Geometry: see drawing. Coordinates: mm, zero at the bounding-box minimum. A direction names the side the tool comes from. Coordinates: 2 decimals unless noted, no trailing zeros. Order: outer loops, then holes, each group sorted by start corner. A loop starts at its lowest first (then second) coordinate and runs counter-clockwise, first axis right, second up.
Item 1: Section D-D on y = 18. Return the cut outline in (x, z).
Item 2: Ray query, line 1 (Y direction, x = 15, z = 3); line 2 (X direction, y = 25.5, z = 16.5); line 3 (Z direction, x = 81, y = 4). Return the intervals inside material, ascending.
Item 3: Mould query, pull axis X, two halves, no side actions, for the marked faces 5, 6 and 7. Classes: released by +X, released by -X, zero draft, split by the parting line, or undercut.
Item 4: Contact query for flat-ended pins moving along their axis: P1, Ø2, axis at y = 6, z = 28.5, coming from the +X side; P2, Ø10.5, axis at x = 15, y = 29, coming from the +Z side; P3, Ø2, axis at y = 30, z = 34.5, coming from the +X side. Output: stop coordinate, or through.
Item 5: Section A-A on y = 10. Return the cut outline in (x, z).
Item 6: Section B-B on z = 9. Return the cut outline in (x, y), then the cut area to 3 significant figures.
Item 7: Section C-C on x = 15. Return the cut outline in (y, z).
Item 8: Reachability of the marked faces 1, 2, 3 and 4 from +Z, -Z, +X, -X, +Y, -Y: full face, straight path, thin tool, end or side. Return the list, or none.
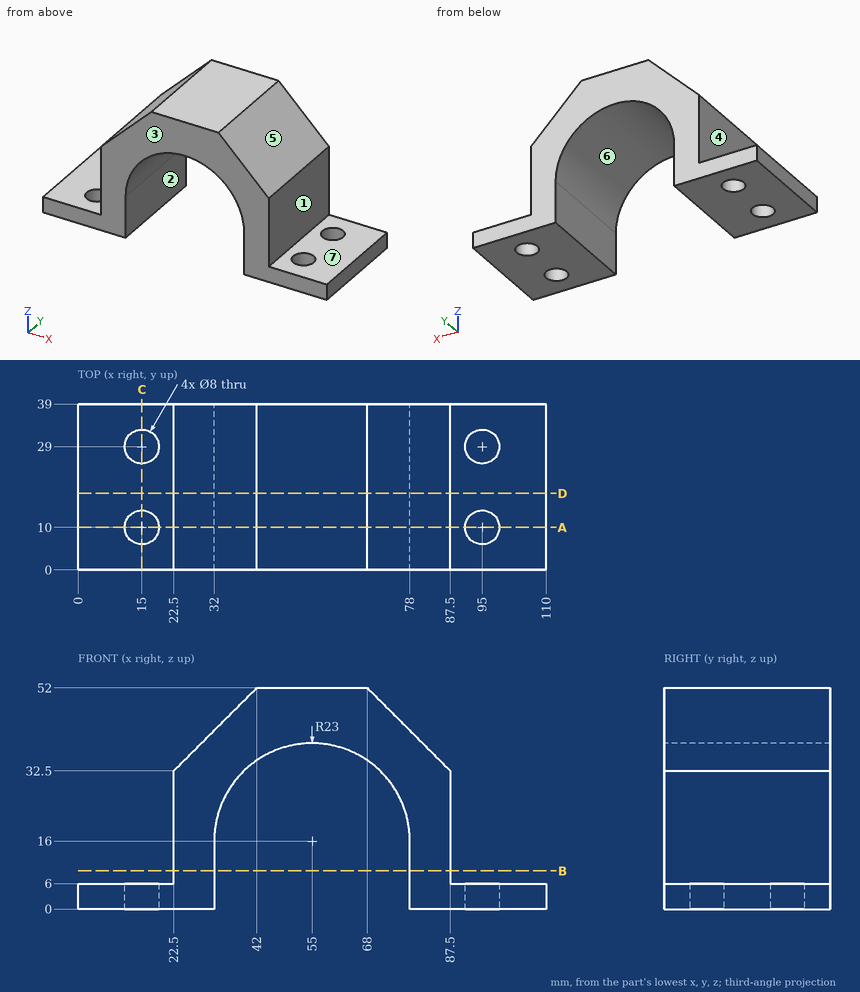
Answer list:
1. outline: (0, 0) - (32, 0) - (32, 16) arc R23 cw to (78, 16) - (78, 0) - (110, 0) - (110, 6) - (87.5, 6) - (87.5, 32.5) - (68, 52) - (42, 52) - (22.5, 32.5) - (22.5, 6) - (0, 6) - close
2. line 1: y = 0 to 6, 14 to 25, 33 to 39
2. line 2: x = 22.5 to 32.01, 77.99 to 87.5
2. line 3: z = 0 to 39
3. face 5: released by +X
3. face 6: undercut
3. face 7: zero draft
4. P1: stops at x = 87.5
4. P2: stops at z = 6
4. P3: stops at x = 86.5
5. outline: (0, 0) - (11, 0) - (11, 6) - (0, 6) - close; (19, 0) - (32, 0) - (32, 16) arc R23 cw to (78, 16) - (78, 0) - (91, 0) - (91, 6) - (87.5, 6) - (87.5, 32.5) - (68, 52) - (42, 52) - (22.5, 32.5) - (22.5, 6) - (19, 6) - close; (99, 0) - (110, 0) - (110, 6) - (99, 6) - close
6. outline: (22.5, 0) - (32, 0) - (32, 39) - (22.5, 39) - close; (78, 0) - (87.5, 0) - (87.5, 39) - (78, 39) - close
6. area: 741 mm2
7. outline: (0, 0) - (6, 0) - (6, 6) - (0, 6) - close; (14, 0) - (25, 0) - (25, 6) - (14, 6) - close; (33, 0) - (39, 0) - (39, 6) - (33, 6) - close
8. face 1: +Z, +X, +Y, -Y
8. face 2: -Z, +Y, -Y
8. face 3: +Z, -Z, +X, -X, -Y
8. face 4: +Z, -X, +Y, -Y
